Read the model definition and answer for the solid it produces. Units are mm, in the model's axes. Face numbers are marked on the shaded views. Give positions to 0.01 mm unless a question says otherwise; leave off trailing zeros. Write each loop counter-clockwise with the first axis right and the second up, starting at its lowest first coordinate (ties: lowest second). Pieces come first, ordered by that corner, then holes. Notation, with made-up numbers: (1.25, 33) -> (50.25, 33) arc R34 ccw to (50.25, 71) -> close; hole circle Ø1 at (-10.75, 37). An arc over 180 degrees is marked (long way). Answer as CSV lines item,"result". Start each with the question number.
1. The part is cut by section B-B, the plane y = 1.15. Determine the outline of the cut face in (x, z).
2. Given pin 1 (4 mm diameter, centred on x = 26.15, z = -8.5, fed in from +Y), flat-ended and moving along its own axis, determine where the tip first touches the part or whether it passes through.
3. For a pull along Y with two mould halves and no side action, classify the marked faces 1 and 2 as pulls with the +Y half, pulls with the -Y half, needs draft (parallel to the pull), parting line crosses it, or undercut.
4. Find the intervals of material crossed by line 1 (Z direction, x = 14.5, y = 1.8); line 2 (Z direction, x = -14, y = 0.8); line 3 (X direction, y = 0.9, z = 23), in increasing order.
from build123d import *

# Parameters (mm, degrees)
SKETCH2_R           = 37.5
SKETCH2_R_2         = 1.75
BOSS_EXTRUDE1_DEPTH = 2
CHAMFER1_SIZE       = 2
FILLET1_R           = 0.5


with BuildPart() as part:
    # Sketch2 → Boss-Extrude1 (new body)
    with BuildSketch(Plane(origin=(0, 0, 0), x_dir=(1, 0, 0), z_dir=(0, 1, 0))):
        with Locations(Location((0, 0, 0), (0, 0, 270))):
            Circle(SKETCH2_R)
        with Locations(Location((0, 27.5, 0), (0, 0, 270))):
            Circle(SKETCH2_R_2, mode=Mode.SUBTRACT)
        with Locations(Location((26.154054198, 8.497967345, 0), (0, 0, 270))):
            Circle(SKETCH2_R_2, mode=Mode.SUBTRACT)
        with Locations(Location((16.164094438, -22.247967345, 0), (0, 0, 270))):
            Circle(SKETCH2_R_2, mode=Mode.SUBTRACT)
        with Locations(Location((-16.164094438, -22.247967345, 0), (0, 0, 270))):
            Circle(SKETCH2_R_2, mode=Mode.SUBTRACT)
        with Locations(Location((-26.154054198, 8.497967345, 0), (0, 0, 270))):
            Circle(SKETCH2_R_2, mode=Mode.SUBTRACT)
    extrude(amount=BOSS_EXTRUDE1_DEPTH)

    # Chamfer1
    chamfer1_edges = [part.edges().sort_by_distance(p)[0] for p in [
        (-26.154054198, 2, -10.247967345),
        (0, 2, -29.25),
        (26.154054198, 2, -10.247967345),
        (16.164094438, 2, 20.497967345),
        (-16.164094438, 2, 20.497967345),
    ]]
    chamfer(chamfer1_edges, length=CHAMFER1_SIZE - 0.0001)  # a hair under: the kernel refuses the full size

    # Fillet1
    fillet1_edges = [part.edges().sort_by_distance(p)[0] for p in [
        (0, 2, -37.5),
    ]]
    fillet(fillet1_edges, radius=FILLET1_R)


solid = part.part
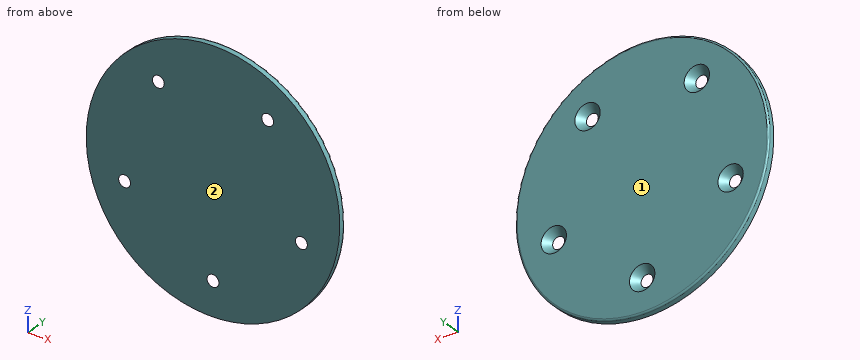
Results found:
1,outline,"circle Ø75 at (0, 0); hole circle Ø5.8 at (-26.15, -8.5); hole circle Ø5.8 at (-16.16, 22.25); hole circle Ø5.8 at (0, -27.5); hole circle Ø5.8 at (16.16, 22.25); hole circle Ø5.8 at (26.15, -8.5)"
2,pin 1,"stops at y = 0.25"
3,face 1,"pulls with the +Y half"
3,face 2,"pulls with the -Y half"
4,line 1,"z = -34.47 to 19.11, 25.38 to 34.47"
4,line 2,"z = -34.79 to 20.9, 23.6 to 34.79"
4,line 3,"x = -29.62 to -18.71, -13.62 to 13.62, 18.71 to 29.62"
